```python
from build123d import *

# Parameters (mm, degrees)
PAH1_SIZE = 0.5


with BuildPart() as part:
    # Çizim1 → Döndür1 (revolve)
    with BuildSketch(Plane.XY, mode=Mode.PRIVATE) as d_nd_r1_sk:
        with BuildLine():
            Line((0, 10), (0, 13))
            Line((0, 13), (-8, 13))
            Line((-8, 13), (-8, 10))
            Line((-8, 10), (-5.732050808, 10))
            ThreePointArc((-5.732050808, 10), (-4, 11), (-2.267949192, 10))
            Line((-2.267949192, 10), (0, 10))
        make_face()
    revolve(d_nd_r1_sk.sketch.rotate(Axis((0, 0, 0), (-1, 0, 0)), 90), axis=Axis((0, 0, 0), (-1, 0, 0)))

    # Pah1
    pah1_edges = [part.edges().sort_by_distance(p)[0] for p in [
        (0, 0, 10),
        (0, 0, 13),
        (-8, 0, 13),
        (-8, 0, 10),
    ]]
    chamfer(pah1_edges, length=PAH1_SIZE)


solid = part.part
```
Verification items for the finished model (mm, model axes). Coordinates: 2 decimals unless noted, no trailing zeros. Write each loop counter-clockwise with the first axis right and the second up, starting at its lowest first coordinate (ties: lowest second). Pieces come first, ordered by that corner, then holes. Notation, with made-up numbers: (-14.5, 53.5) - (35.5, 53.5) arc R21 cw to (35.5, 83.5) - close; hole circle Ø10 at (-25.5, -18). An arc over 180 degrees is marked (long way). Write item = value, one per line.
Q1. Mould release check, pull along Z, two halves, no side actions. Record for faces 1 (the face through (-4.049, 7.91, 10.316)), 2 (the face through (-7, 0, 10)): released by +Z, released by -Z, zero draft, split by the parting line, or undercut.
Answer:
face_1 = split by the parting line
face_2 = undercut
Q2. Go/stop test with flat-tipped pins: pin 1 Ø3 at (x, z) = (-2.5, -3) entering from -Y; pin 2 Ø12 at (y, z) = (-5, 1.5) entering from +X; pin 3 Ø1 at (x, z) = (-4.5, 7.5) entering from -Y; pin 4 Ø4 at (x, z) = (-2, 7) entering from -Y. Record where each tip stops, or that it passes through.
Answer:
pin_1 = -12.91
pin_2 = 0
pin_3 = -10.95
pin_4 = -12
Q3. Material ranges on L1, parallel to Y at x = -6.4, z = 0; L2, parallel to Z at x = -1.75, y = 5; L3, parallel to Z at x = -3.25, y = -7.75, recorded low to high. Write a range as from..to.
Answer:
L1 = -13..-10, 10..13
L2 = -12..-8.66, 8.66..12
L3 = -10.44..-7.6, 7.6..10.44
Q4. Cross-section at C-C (x = -2.75). Enter the section's corners in (y, z), plus the area to 3 significant figures.
Answer:
outline = circle Ø26 at (0, 0); hole circle Ø21.12 at (0, 0)
area = 181 mm²
Q5. Cross-section at D-D (x = -5). Enter the section's corners in (y, z), plus the area to 3 significant figures.
Answer:
outline = circle Ø26 at (0, 0); hole circle Ø21.46 at (0, 0)
area = 169 mm²
Q6. Cross-section at A-A (z = 0). Enter the section's corners in (x, y).
Answer:
outline = (-8, -12.5) - (-7.5, -13) - (-0.5, -13) - (0, -12.5) - (0, -10.5) - (-0.5, -10) - (-2.27, -10) arc R2 cw to (-5.73, -10) - (-7.5, -10) - (-8, -10.5) - close; (-8, 10.5) - (-7.5, 10) - (-5.73, 10) arc R2 cw to (-2.27, 10) - (-0.5, 10) - (0, 10.5) - (0, 12.5) - (-0.5, 13) - (-7.5, 13) - (-8, 12.5) - close
